Autodesk Inventor part; units mm, degrees
ref_plane "YZ Plane" through (0, 0, 0) normal (1, 0, 0) x (0, 1, 0)
ref_plane "XZ Plane" through (0, 0, 0) normal (0, 1, 0) x (-1, 0, 0)
ref_plane "XY Plane" through (0, 0, 0) normal (0, 0, 1) x (1, 0, 0)
sketch "Sketch1" plane through (0, 0, 0) normal (0, 1, 0) x (-1, 0, 0)
  line L0 (0, 0) -> (0, -230.652) construction
  line L1 (5, 0) -> (5, -230.652)
  line L2 (-5, -230.652) -> (-5, 0)
  arc A0 (5, 0) -> (-5, 0) centre (0, 0) ccw
  arc A1 (-5, -230.652) -> (5, -230.652) centre (0, -230.652) ccw
  circle A2 centre (0, 0) radius 1.65
  circle A3 centre (0, -230.652) radius 1.65
  arc A4 (-5, -230.652) -> (-5, 0) centre (-897.5805, -115.326) ccw
  arc A5 (5, -230.652) -> (5, 0) centre (-887.5805, -115.326) ccw
  point P0 (0, -115.326)
  dimension "d0" = 3.3
  dimension "d1" = 3.3
  dimension "d2" = 10
  dimension "d3" = 230.652
  dimension "d14" = 900
  dimension "d15" = 900
extrude "Extrusion1" add sketch "Sketch1" along normal blind 3 contours A5 L1 | L1 A1 A4 A0
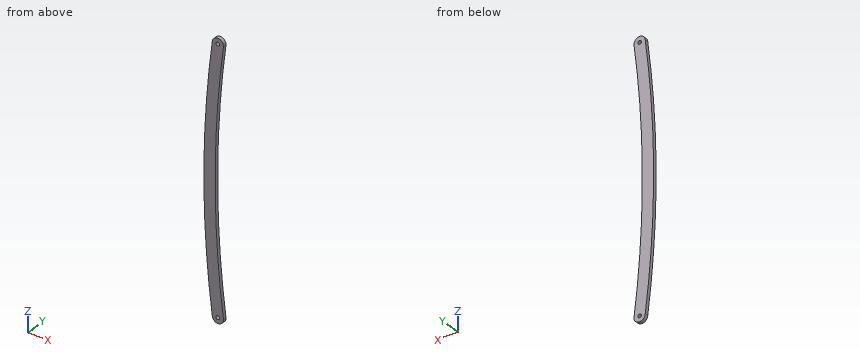
CAD build for the part. Positions are in the model's coordinates, mm. Round coordinates to 2 decimals unless told otherwise and drop trailing zeros. Write each loop counter-clockwise with the first axis right and the second up, starting at its lowest first coordinate (ties: lowest second). Pieces come first, ordered by that corner, then holes.
Item 1: Drop flat-ended pins along their axis: pin 1 Ø1 at (y, z) = (2, -59) entering from +X; pin 2 Ø1 at (y, z) = (2.5, -141.5) entering from +X; pin 3 Ø3 at (x, z) = (0, -230.652) entering from -Y; pin 4 Ø6 at (x, z) = (2, -38) entering from -Y. Give the stop position or say it passes through.
Filled in:
pin 1: stops at x = -0.62
pin 2: stops at x = -2.02
pin 3: passes through
pin 4: stops at y = 0
Item 2: Band-saw the part on A-A on y = 2.1. Write the cut outline in (x, z).
Filled in:
outline: (-5, -230.65) arc R5 ccw to (5, -230.65) arc R900 cw to (5, 0) arc R5 ccw to (-5, 0) arc R900 ccw to start; hole circle Ø3.3 at (0, -230.65); hole circle Ø3.3 at (0, 0)
Item 3: Band-saw the part on C-C on z = -62.5. Write the cut outline in (x, y).
Filled in:
outline: (-10.87, 0) - (-0.87, 0) - (-0.87, 3) - (-10.87, 3) - close
Item 4: Drill centre lines: L1, parallel to X at y = 2.55, z = -113.5; L2, parallel to Z at x = -4, y = 1.35; L3, parallel to X at y = 2.5, z = -163. Where is each one in solid material? Low to high.
Filled in:
L1: x = -12.42 to -2.42
L2: z = -233.65 to 3
L3: x = -11.16 to -1.16
